Input: part model. Units: mm. Frame: model coordinates. A direction names the side the tool comes from. Coordinates: 2 decimals unless noted, no trailing zeros. Loops run counter-clockwise (first coordinate to the right, second up) from the corner with the lowest first, then second, coordinate; pieces in that order, holes last. Notation, with made-up numbers: (-2, 25.25) - (37, 25.25) arc R17 cw to (37, 52.25) - close; hole circle Ø1 at (76.5, -29). An arc over 180 degrees is marked (long way). Use one line per item in the form item = value.
from build123d import *

# Parameters (mm, degrees)
SKETCH_1_W      = 42.2
SKETCH_1_H      = 42.2
SKETCH_1_W_2    = 40.2
SKETCH_1_H_2    = 40.2
EXTRUDE_1_DEPTH = 4
CHAMFER_1_SIZE  = 3.9
CHAMFER_2_SIZE  = 4.2


with BuildPart() as part:
    # 草图1 → 凸台-拉伸1 (new body)
    with BuildSketch(Plane(origin=(0, 0, 0), x_dir=(1, 0, 0), z_dir=(0, 1, 0))):
        with Locations((20.1, 20.1)):
            Rectangle(SKETCH_1_W, SKETCH_1_H)
        with Locations((20.1, 20.1)):
            Rectangle(SKETCH_1_W_2, SKETCH_1_H_2, mode=Mode.SUBTRACT)
    extrude(amount=EXTRUDE_1_DEPTH)

    # 倒角1
    chamfer_1_edges = [part.edges().sort_by_distance(p)[0] for p in [
        (0, 2, -40.2),
        (0, 2, 0),
        (40.2, 2, 0),
        (40.2, 2, -40.2),
    ]]
    chamfer(chamfer_1_edges, length=CHAMFER_1_SIZE)

    # 倒角2
    chamfer_2_edges = [part.edges().sort_by_distance(p)[0] for p in [
        (-1, 2, 1),
        (-1, 2, -41.2),
        (41.2, 2, -41.2),
        (41.2, 2, 1),
    ]]
    chamfer(chamfer_2_edges, length=CHAMFER_2_SIZE)


solid = part.part
Q1. Set-up query: faces 4 (the flat face through (40.2, 2, -20)), 5 (the flat face through (-1, 2, -20)). Return all of +Z, -Z, +X, -X, +Y, -Y with unobstructed straight access to the full face (end or side cutting, diameter ignored); none if empty.
Check values:
face_4 = +Y, -Y
face_5 = +Z, -Z, -X, +Y, -Y
Q2. Ray query, line 1 along Z through (x, y) = (7.5, 1.55); line 2 along X through (y, z) = (2.9, -19); line 3 along Z through (x, y) = (39, 3.25). Return the intervals inside material, ascending. Write a range as [from, to].
Check values:
line_1 = [-41.2, -40.2], [0, 1]
line_2 = [-1, 0], [40.2, 41.2]
line_3 = [-39.2, -37.5], [-2.7, -1]
Q3. Cut plane A-A, the plane x = 9. Return loops of the section in (y, z), then the cut area to 3 significant figures.
Check values:
outline = (0, -41.2) - (4, -41.2) - (4, -40.2) - (0, -40.2) - close; (0, 0) - (4, 0) - (4, 1) - (0, 1) - close
area = 8.00 mm²
Q4. Pull-direction query (X, two-part tool) for faces 1 (the flat face through (20, 2, -41.2)), 2 (the flat face through (0, 2, -20)), 3 (the flat face through (41.2, 2, -20)); classes: pulls with the +X half, pulls with the -X half, needs draft (parallel to the pull), parting line crosses it, or undercut.
Check values:
face_1 = needs draft
face_2 = undercut
face_3 = pulls with the +X half
Q5. Cut plane B-B, the plane z = -18.5. Return loops of the section in (x, y).
Check values:
outline = (-1, 0) - (0, 0) - (0, 4) - (-1, 4) - close; (40.2, 0) - (41.2, 0) - (41.2, 4) - (40.2, 4) - close
Q6. Cut plane C-C, the plane y = 2.35. Return loops of the section in (x, z), then the cut area to 3 significant figures.
Check values:
outline = (-1, -37) - (3.2, -41.2) - (37, -41.2) - (41.2, -37) - (41.2, -3.2) - (37, 1) - (3.2, 1) - (-1, -3.2) - close; hole (0, -36.3) - (3.9, -40.2) - (36.3, -40.2) - (40.2, -36.3) - (40.2, -3.9) - (36.3, 0) - (3.9, 0) - (0, -3.9) - close
area = 160 mm²
